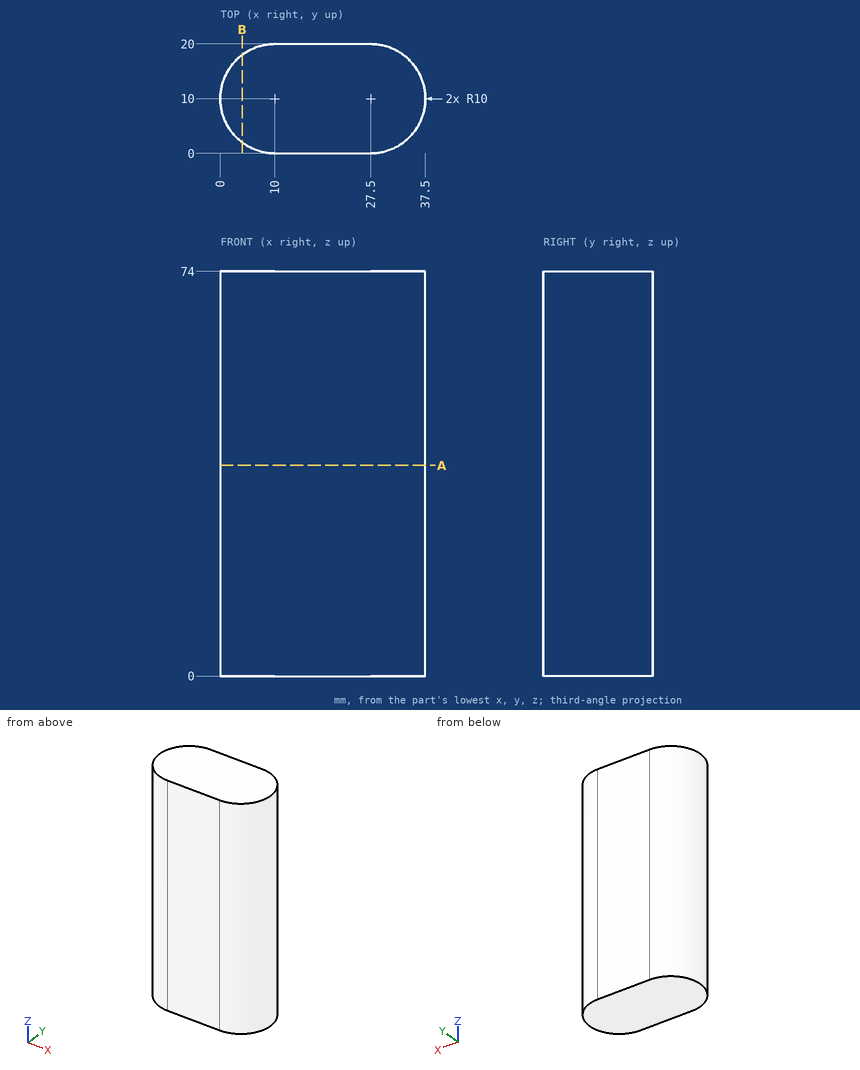
Could you check a few things on this drawing? It's one solid part, dimensions in mm from its lowest x, y, z. Coordinates: 2 decimals unless noted, no trailing zeros. Order: outer loops, then holes, each group sorted by start corner. A loop starts at its lowest first (then second) coordinate and runs counter-clockwise, first axis right, second up. Notation, with made-up numbers: (59, -37.5) - (79, -37.5) arc R20 ccw to (79, -20.5) - close; hole circle Ø8 at (9.5, 23.25). An arc over 180 degrees is marked (long way). One line per question, with ' | ' between items.
(1) If I drill on L1, parallel to Y at x = 36.5, z = 3.5; L2, parallel to X at y = 14, z = 37.5; L3, parallel to X at y = 2, z = 26, over which ranges is the centre line in solid material (lowest first)?
Report:
L1: y = 5.64 to 14.36 | L2: x = 0.83 to 36.67 | L3: x = 4 to 33.5
(2) Will these pins go through, and if not, where does the flat tip stop? pin 1 (5 mm diameter, centred on x = 29.5, z = 20, fed in from -Y); pin 2 (1 mm diameter, centred on x = 30.5, z = 50.5, fed in from +Y); pin 3 (5 mm diameter, centred on x = 6.5, z = 37, fed in from -Y); pin 4 (5 mm diameter, centred on y = 13, z = 31.5, fed in from +X).
Report:
pin 1: stops at y = 0 | pin 2: stops at y = 19.68 | pin 3: stops at y = 0.05 | pin 4: stops at x = 37.49
(3) Suppose I cut it at A-A on z = 38.5. List the corners of the cut face in (x, y) for me.
Report:
outline: (10, 0) - (27.5, 0) arc R10 ccw to (27.5, 20) - (10, 20) arc R10 ccw to start
(4) Suppose I cut it at B-B on x = 4. List the corners of the cut face in (y, z) for me.
Report:
outline: (2, 0) - (18, 0) - (18, 74) - (2, 74) - close
